```python
from build123d import *

# Parameters (mm, degrees)
SKETCH001_W   = 16
SKETCH001_H   = 3
SKETCH001_W_2 = 0.9
SKETCH001_H_2 = 7
PAD_DEPTH     = 22
SKETCH_R      = 0.7
PAD001_DEPTH  = 3.5
SKETCH002_R   = 1.25
HOLE_DEPTH    = 5.001


with BuildPart() as body001:
    # Sketch001 → Pad (new body)
    with BuildSketch(Plane.XY):
        with Locations((8, 0)):
            Rectangle(SKETCH001_W, SKETCH001_H)
        with Locations((15.55, 0)):
            Rectangle(SKETCH001_W_2, SKETCH001_H_2)
        with Locations((12.516667, 0)):
            Rectangle(SKETCH001_W_2, SKETCH001_H_2)
        with Locations((6.45, 0)):
            Rectangle(SKETCH001_W_2, SKETCH001_H_2)
        with Locations((9.483333, 0)):
            Rectangle(SKETCH001_W_2, SKETCH001_H_2)
    extrude(amount=PAD_DEPTH)


with BuildPart() as pin:
    # Sketch → Pad001 (new body)
    with BuildSketch(Plane.XY):
        with Locations((14.7, 0)):
            Circle(SKETCH_R)
    extrude(amount=-PAD001_DEPTH)

    # Boolean: union Body001
    add(body001.part)

    # Mirrored: Pin across YZ


with BuildPart() as pin_1:
    add(pin.part)
    add(pin.part.mirror(Plane.YZ))

    # Sketch002 (on Face65 of Mirrored) → Hole (cut, through all)
    with BuildSketch(Plane.XZ.offset(1.5)):
        with Locations((0, 18)):
            Circle(SKETCH002_R)
    extrude(amount=-HOLE_DEPTH, mode=Mode.SUBTRACT)


solid = pin_1.part
```
Model file for the job. Use its own axes, mm. A direction names the side the tool comes from. Round coordinates to 2 decimals unless told otherwise and drop trailing zeros. Write each loop counter-clockwise with the first axis right and the second up, starting at its lowest first coordinate (ties: lowest second). Pieces come first, ordered by that corner, then holes. Notation, with made-up numbers: (44, -6) -> (72, -6) arc R25 ccw to (72, 11) -> close; hole circle Ø3 at (26.5, -2). An arc over 180 degrees is marked (long way). Answer as CSV lines item,"result".
1. Mould opens along X. For faces 1 (the face through (-8, 1.5, 11)), 2 (the face through (15, 0, -3.5)), 3 (the face through (12.067, 2, 11)) say: +X half, -X half, draft (parallel to the pull), parting line (faces both ways), or undercut.
Resolved:
face 1,"undercut"
face 2,"draft"
face 3,"undercut"
2. Pin check, flat tips, straight feed: pin 1 Ø2 at (x, z) = (7, 2.5) entering from -Y; pin 2 Ø2 at (x, y) = (3.5, 1.5) entering from -Z. Stop position of each tip, or through.
Resolved:
pin 1,"y = -3.5"
pin 2,"z = 0"
3. Drill centre lines: line 1 (Z direction, x = 0, y = 0.75); line 2 (Y direction, x = -11.5, z = 14); line 3 (Z direction, x = 9.5, y = -1). Where is each one in solid material? Low to high.
Resolved:
line 1,"0 to 16.75, 19.25 to 22"
line 2,"-1.5 to 1.5"
line 3,"0 to 22"
4. Slice it at D-D, the plane x = -14.7. List the corners of the cut face in (y, z), plus the area to 3 significant figures.
Resolved:
outline,"(-1.5, 0) -> (-0.7, 0) -> (-0.7, -3.5) -> (0.7, -3.5) -> (0.7, 0) -> (1.5, 0) -> (1.5, 22) -> (-1.5, 22) -> close"
area,"70.9 mm²"
5. Slice it at B-B, the plane y = -2. State how many separate pieces and enclosed holes the cut face has, plus the area to 3 significant figures.
Resolved:
separate pieces,"8"
enclosed holes,"0"
area,"158 mm²"
6. Slice it at A-A, the plane x = 0. List the corners of the cut face in (y, z).
Resolved:
outline,"(-1.5, 0) -> (1.5, 0) -> (1.5, 16.75) -> (-1.5, 16.75) -> close; (-1.5, 19.25) -> (1.5, 19.25) -> (1.5, 22) -> (-1.5, 22) -> close"
7. Tool access for faces 4 (the face through (-9.033, -3, 11)), 5 (the face through (12.967, 2, 11)), 6 (the face through (-15.347, -0.268, -1.726)): list every direction of +Z, -Z, +X, -X, +Y, -Y with a clear straight run to the whole face (end or side of a thin tool).
Resolved:
face 4,"+Z, -Z, -Y"
face 5,"+Z, -Z, +Y"
face 6,"-Z"
8. Slice it at C-C, the plane y = 0. List the corners of the cut face in (x, z), plus the area to 3 significant figures.
Resolved:
outline,"(-16, 0) -> (-15.4, 0) -> (-15.4, -3.5) -> (-14, -3.5) -> (-14, 0) -> (14, 0) -> (14, -3.5) -> (15.4, -3.5) -> (15.4, 0) -> (16, 0) -> (16, 22) -> (-16, 22) -> close; hole circle Ø2.5 at (0, 18)"
area,"709 mm²"
